from build123d import *

# Parameters (mm, degrees)
SKETCH1_R           = 75
SKETCH1_R_2         = 51.2
BOSS_EXTRUDE1_DEPTH = 4
SKETCH2_R           = 2.25
SKETCH2_R_2         = 1
CUT_EXTRUDE1_DEPTH  = 107.141415103
CIRPATTERN1_COUNT   = 9
SKETCH3_R           = 6.25
CUT_EXTRUDE2_DEPTH  = 10


with BuildPart() as part:
    # Sketch1 → Boss-Extrude1 (new body)
    with BuildSketch(Plane(origin=(0, 0, 0), x_dir=(1, 0, 0), z_dir=(0, 1, 0))):
        with Locations(Location((0, 0, 0), (0, 0, 270))):
            Circle(SKETCH1_R)
        with Locations(Location((0, 0, 0), (0, 0, 270))):
            Circle(SKETCH1_R_2, mode=Mode.SUBTRACT)
    extrude(amount=BOSS_EXTRUDE1_DEPTH)

    # Sketch2 → Cut-Extrude1 (cut, through all)
    with BuildSketch(Plane(origin=(0, 4, 0), x_dir=(1, 0, 0), z_dir=(0, 1, 0))):
        with Locations(Location((0, 66, 0), (0, 0, 270))):
            Circle(SKETCH2_R)
        with Locations(Location((4.246572956, 69.876740658, 0), (0, 0, 270))):
            Circle(SKETCH2_R_2)
        with Locations(Location((4.246572956, 62.123259342, 0), (0, 0, 270))):
            Circle(SKETCH2_R_2)
        with Locations(Location((-4.246572956, 62.123259342, 0), (0, 0, 270))):
            Circle(SKETCH2_R_2)
        with Locations(Location((-4.246572956, 69.876740658, 0), (0, 0, 270))):
            Circle(SKETCH2_R_2)
    cut_extrude1 = extrude(amount=-CUT_EXTRUDE1_DEPTH, mode=Mode.SUBTRACT)

    # CirPattern1: Cut-Extrude1 ×9 about axis
    cirpattern1_axis = Axis((0, 0, 0), (0, 1, 0))
    for i in range(1, CIRPATTERN1_COUNT):
        add(cut_extrude1.rotate(cirpattern1_axis, i * 360 / CIRPATTERN1_COUNT), mode=Mode.SUBTRACT)

    # Sketch3 → Cut-Extrude2 (cut)
    with BuildSketch(Plane(origin=(0, 4, 0), x_dir=(1, 0, 0), z_dir=(0, 1, 0))):
        with Locations((0, 66)):
            Circle(SKETCH3_R)
    extrude(amount=-CUT_EXTRUDE2_DEPTH, mode=Mode.SUBTRACT)


solid = part.part
Part model, mm, in its own coordinate system. A direction names the side the tool comes from. Round coordinates to 2 decimals unless told otherwise and drop trailing zeros. Loops run counter-clockwise (first coordinate to the right, second up) from the corner with the lowest first, then second, coordinate; pieces in that order, holes last. Notation, with made-up numbers: (-21, -12.75) - (-5, -12.75) arc R11 cw to (-5, 8.25) - close; hole circle Ø8 at (34.25, 47.25). An arc over 180 degrees is marked (long way). Answer as a JSON object with one key per item and string values.
Item 1: Pull direction X, two halves, no side cores. Call faces 3 (the face through (-45.636, 1.972, -59.517)), 4 (the face through (-0.06, 2.03, -59.75)), 5 (the face through (-16, 4, 49)): pulls with the +X half, pulls with the -X half, needs draft (parallel to the pull), parting line crosses it, or undercut.
Output:
{"face 3": "parting line crosses it", "face 4": "undercut", "face 5": "needs draft"}
Item 2: Band-saw the part on C-C on y = 2.2. State how many separate pieces and enclosed holes the cut face has, plus the area to 3 significant figures.
Output:
{"separate pieces": "1", "enclosed holes": "42", "area": "9,080 mm2"}
Item 3: Band-saw the part on A-A on z = 0. List the corners of the cut face in (x, y).
Output:
{"outline": "(-75, 0) - (-51.2, 0) - (-51.2, 4) - (-75, 4) - close; (51.2, 0) - (75, 0) - (75, 4) - (51.2, 4) - close"}
Item 4: Band-saw the part on B-B on x = 0. List the corners of the cut face in (y, z), plus the area to 3 significant figures.
Output:
{"outline": "(0, -75) - (4, -75) - (4, -72.25) - (0, -72.25) - close; (0, -59.75) - (4, -59.75) - (4, -51.2) - (0, -51.2) - close; (0, 51.2) - (4, 51.2) - (4, 75) - (0, 75) - close", "area": "140 mm2"}
Item 5: Pin check, flat tip, straight feed: pin 1 (1 mm diameter, centred on y = 2.5, z = -28, fed in from -X). Stop position of the tip, or through.
Output:
{"pin 1": "x = -69.78"}
Item 6: Tool access for faces 1 (the face through (-6.25, 2.03, -66.05)), 2 (the face through (-16, 0, 49)): list every direction of +Z, -Z, +X, -X, +Y, -Y with a clear straight run to the whole face (end or side of a thin tool).
Output:
{"face 1": "+Y, -Y", "face 2": "+Z, -Z, +X, -X, -Y"}
Item 7: Wall check: L1, parallel to Z at x = -0.5, y = 0.95; L2, parallel to X at y = 3.75, z = -45.5; L3, parallel to Z at x = -41, y = 0.3. Give the ranges that are in metal, low to high.
Output:
{"L1": "-75 to -72.23, -59.77 to -51.2, 51.2 to 75", "L2": "-59.62 to -43.95, -42.42 to -23.48, 23.48 to 42.42, 43.95 to 59.62", "L3": "-62.8 to -57.01, -55.51 to -52.3, -48.82 to -30.67, 30.67 to 62.8"}
